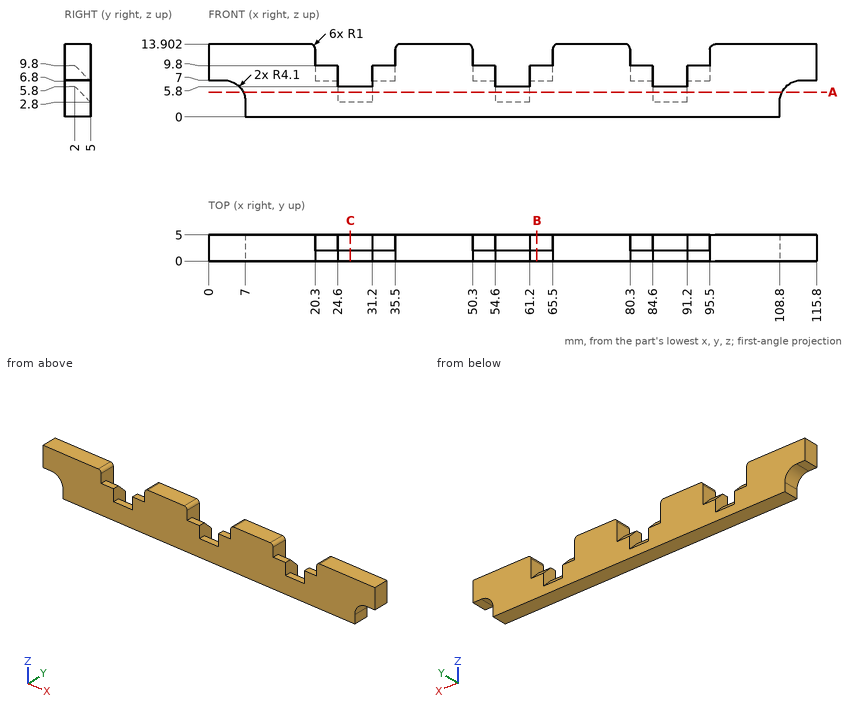
Part print with two shaded views. Sizes in mm from the minimum x, y, z corner. Coordinates: 2 decimals unless noted, no trailing zeros. Write each loop counter-clockwise with the first axis right and the second up, starting at its lowest first coordinate (ties: lowest second). Pieces come first, ordered by that corner, then holes. Notation, with made-up numbers: (-15, 19.25) - (15, 19.25) arc R8 ccw to (15, 29.25) - close; hole circle Ø9 at (39, -31). An arc over 180 degrees is marked (long way). Use a Markdown table: item, result. Add a question column.
Item 1: Band-saw the part on A-A, the plane z = 4.75. Write the cut outline in (x, y).
Item 2: Band-saw the part on B-B, the plane x = 62.5. Write the cut outline in (y, z).
Item 3: Drill centre lines: line 1 along X through (y, z) = (0.5, 11); line 2 along X through (y, z) = (2.6, 7.5); line 3 along X through (y, z) = (1.1, 2). Where is each one in solid material? Low to high.
Item 4: Drop flat-ended pins along their axis: pin 1 (2 mm diameter, centred on x = 21.5, y = 0.5, fed in from +Z); pin 2 (1.5 mm diameter, centred on y = 3, z = 5.5, fed in from +X) (1 decimal); pin 3 (0.9 mm diameter, centred on y = 2.5, z = 1.5, fed in from -X). Give the stop position or say it passes through.
Item 5: Band-saw the part on C-C, the plane x = 27. Write the cut outline in (y, z).
A:
| question | item | result |
|---|---|---|
| 1 | outline | (6.56, 0) - (109.24, 0) - (109.24, 5) - (91.2, 5) - (91.2, 3.05) - (84.6, 3.05) - (84.6, 5) - (61.2, 5) - (61.2, 3.05) - (54.6, 3.05) - (54.6, 5) - (31.2, 5) - (31.2, 3.05) - (24.6, 3.05) - (24.6, 5) - (6.56, 5) - close |
| 2 | outline | (0, 0) - (5, 0) - (5, 6.8) - (2, 9.8) - (0, 9.8) - close |
| 3 | line 1 | x = 0 to 20.3, 35.5 to 50.3, 65.5 to 80.3, 95.5 to 115.8 |
| 3 | line 2 | x = 0 to 24.6, 31.2 to 54.6, 61.2 to 84.6, 91.2 to 115.8 |
| 3 | line 3 | x = 7 to 108.8 |
| 4 | pin 1 | stops at z = 9.8 |
| 4 | pin 2 | stops at x = 110.5 |
| 4 | pin 3 | stops at x = 7 |
| 5 | outline | (0, 0) - (5, 0) - (5, 2.8) - (2, 5.8) - (0, 5.8) - close |
